Could you check a few things on this model? Use its own coordinates, in mm. Face numbers are marked on the shaded views. A direction names the side the tool comes from. Give positions to 0.01 mm unless a question says otherwise; leave off trailing zeros. Loops run counter-clockwise (first coordinate to the right, second up) from the corner with the lowest first, then second, coordinate; pieces in that order, holes last. Notation, with made-up numbers: (8.5, 55.5) -> (43.5, 55.5) arc R33 cw to (43.5, 83.5) -> close; hole circle Ø6 at (7.5, -23). An arc over 180 degrees is marked (long way). Put each result on its own line as item: value.
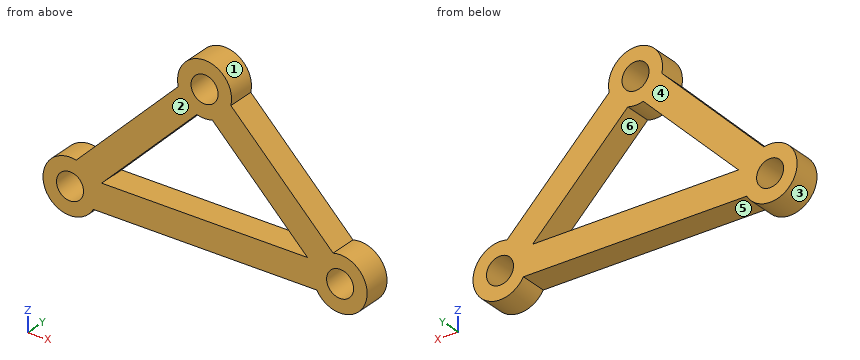
```python
from build123d import *

# Parameters (mm, degrees)
BOSS_EXTRUDE1_DEPTH   = 5
F_5_0MM_DOWEL_HOLE1_D = 5


with BuildPart() as part:
    # Sketch2 → Boss-Extrude1 (new body)
    with BuildSketch(Plane(origin=(0, 0, 0), x_dir=(1, 0, 0), z_dir=(0, 1, 0))):
        with BuildLine():
            Line((-32.269872981, 20.929032067), (9.069872981, 20.929032067))
            ThreePointArc((9.069872981, 20.929032067), (18.019397663, 20.342449229), (12.105904774, 13.599402936))
            Line((12.105904774, 13.599402936), (-6.82412184, -5.330623679))
            ThreePointArc((-6.82412184, -5.330623679), (-11.690092491, -11.4805496), (-16.556063141, -5.330623679))
            Line((-16.556063141, -5.330623679), (-35.449810526, 13.563123706))
            ThreePointArc((-35.449810526, 13.563123706), (-41.190492208, 20.410794235), (-32.269872981, 20.929032067))
        make_face()
        with BuildLine():
            Line((-30.744651075, 15.929032067), (7.364466094, 15.929032067))
            Line((7.364466094, 15.929032067), (-10.255377332, -1.690811359))
            ThreePointArc((-10.255377332, -1.690811359), (-11.690092491, -1.4805496), (-13.124807649, -1.690811359))
            Line((-13.124807649, -1.690811359), (-30.744651075, 15.929032067))
        make_face(mode=Mode.SUBTRACT)
    extrude(amount=BOSS_EXTRUDE1_DEPTH)

    # Ø5.0mm Dowel Hole1 (through all)
    with Locations(Plane(origin=(0, 5, 0), x_dir=(1, 0, 0), z_dir=(0, 1, 0))):
        with Locations((13.4, 18.429032067), (-36.6, 18.429032067), (-11.690092491, -6.4805496)):
            Hole(F_5_0MM_DOWEL_HOLE1_D / 2)


solid = part.part
```
1. If we section it at B-B (y = 2.9): List the corners of the cut face in (x, z) for me.
Recorded:
outline: (-35.45, -13.56) arc R5 ccw (long way) to (-32.27, -20.93) -> (9.07, -20.93) arc R5 ccw (long way) to (12.11, -13.6) -> (-6.82, 5.33) arc R5 ccw (long way) to (-16.56, 5.33) -> close; hole circle Ø5 at (-36.6, -18.43); hole (-30.74, -15.93) -> (7.36, -15.93) -> (-10.26, 1.69) arc R5 cw to (-13.12, 1.69) -> close; hole circle Ø5 at (-11.69, 6.48); hole circle Ø5 at (13.4, -18.43)
2. I'm going to push flat-ended pins straight in: pin 1 (2.5 mm diameter, centred on x = -14.5, y = 2, fed in from +Z); pin 2 (4.5 mm diameter, centred on x = 13.4, z = -18.43, fed in from +Y); pin 3 (6.5 mm diameter, centred on x = -11.69, z = 6.48, fed in from -Y); pin 4 (2 mm diameter, centred on x = -30, y = 2.5, fed in from -Z). Where does each tip first touch, or does it pass through?
Recorded:
pin 1: stops at z = 11.23
pin 2: passes through
pin 3: stops at y = 0
pin 4: stops at z = -20.93
3. If we section it at C-C (z = -2.5): List the corners of the cut face in (x, y) for me.
Recorded:
outline: (-24.39, 0) -> (-17.32, 0) -> (-17.32, 5) -> (-24.39, 5) -> close; (-6.06, 0) -> (1.01, 0) -> (1.01, 5) -> (-6.06, 5) -> close
4. I need wall thicknesses on line 1 (Z direction, x = 13.4, y = 1.6); line 2 (X direction, y = 2.1, z = -19.5); line 3 (Z direction, x = -22, y = 3). Which ranges of each line are inside material? Lowest first, please.
Recorded:
line 1: z = -23.43 to -20.93, -15.93 to -13.43
line 2: x = -41.48 to -38.86, -34.34 to 11.14, 15.66 to 18.28
line 3: z = -20.93 to -15.93, -7.18 to -0.11
5. If we section it at A-A (x = -36.6): List the corners of the cut face in (y, z) for me.
Recorded:
outline: (0, -23.43) -> (5, -23.43) -> (5, -20.93) -> (0, -20.93) -> close; (0, -15.93) -> (5, -15.93) -> (5, -13.43) -> (0, -13.43) -> close
6. For the marked faces 4, 5 and 6, which set-ups out of +Z, -Z, +X, -X, +Y, -Y let a thin tool reach every point of the face, with its end or its side?
Recorded:
face 4: +Z, -Z, +X, -X, +Y
face 5: -Z, +Y, -Y
face 6: +Y, -Y
7. Thinking about a two-plate mould opening in X: for the marked faces 1, 2 and 3, which applies, pulls with the +X half, pulls with the -X half, needs draft (parallel to the pull), parting line crosses it, or undercut?
Recorded:
face 1: parting line crosses it
face 2: needs draft
face 3: undercut
